Geometry check sheet. Reference: the model listing, model coordinates, mm. A direction names the side the tool comes from. Round coordinates to 2 decimals unless told otherwise and drop trailing zeros. Write each loop counter-clockwise with the first axis right and the second up, starting at its lowest first coordinate (ties: lowest second). Pieces come first, ordered by that corner, then holes. Notation, with made-up numbers: M 32.25,-11.75 L 83.25,-11.75 A12 ccw 83.25,-5.75 Z; hole C 83,20 d4. An arc over 180 degrees is marked long. Put each result on its own line as item: value. Start each with the question number.
(1) Mould release check, pull along X, two halves, no side actions. Record for faces 3 (the flat face through (-63.493, 124.331, 0.986)), 4 (the flat face through (2, 44, 0)), 5 (the cylindrical face through (48.25, 61.87, 1.01)): pulls with the +X half, pulls with the -X half, needs draft (parallel to the pull), parting line crosses it, or undercut.
(2) Material ranges on probe 1 along X at (y, z) = (14.5, 0.7); probe 2 along Y at (x, z) = (110, 1.2); probe 3 along Y at (x, z) = (91.5, 0.1), recorded low to high.
(3) Tool access check on faces 1 (the cylindrical face through (-48.25, 61.87, 1.01)), 2 (the flat face through (2, 44, 2)). Record the directions out of +Z, -Z, +X, -X, +Y, -Y that give a thin tool (end or side, any length) a straight path to the whole face; none if there is none.
(4) Section check B-B on z = 0.8. Count the separate pieces of the cut face and the enclosed holes in it, then the cut area to 3 significant figures.
(5) Gauge pin test, flat ends, axial feed: pin 1 (1 mm diameter, centred on x = -126, z = 1, fed in from +Y); pin 2 (1 mm diameter, centred on y = 107, z = 1.5, fed in from +X). Record the tip position at first contact, or that the pin passes through.
(6) Section check A-A on x = -18.5. Record the cut outline in (y, z).
from build123d import *

# Parameters (mm, degrees)
SKETCH1_W           = 20
SKETCH1_H           = 2.2
BOSS_EXTRUDE1_DEPTH = 2
FILLET1_R           = 10
SKETCH2_R           = 2.1
CUT_EXTRUDE1_DEPTH  = 5


with BuildPart() as part:
    # Sketch1 → Boss-Extrude1 (new body)
    with BuildSketch(Plane.XY):
        Polygon((125.000000001, -10.433333333), (-124.999999999, -10.433333333), (-124.999999999, 19.566666667), (-127.199999999, 19.566666667), (-127.199999999, 39.566666667), (-124.999999999, 39.566666667), (-124.999999999, 129.566666667), (-127.199999999, 129.566666667), (-127.199999999, 149.566666667), (-124.999999999, 149.566666667), (-124.999999999, 179.566666667), (-74.999999999, 179.566666667), (-50, 59.566666667), (50, 59.566666667), (75.000000001, 179.566666667), (125.000000001, 179.566666667), (125.000000001, 149.566666667), (127.200000001, 149.566666667), (127.200000001, 129.566666667), (125.000000001, 129.566666667), (125.000000001, 39.566666667), (127.200000001, 39.566666667), (127.200000001, 19.566666667), (125.000000001, 19.566666667), align=None)
        with Locations((85.000000001, -2.933333333)):
            Rectangle(SKETCH1_W, SKETCH1_H, mode=Mode.SUBTRACT)
        with Locations((-84.999999999, -2.933333333)):
            Rectangle(SKETCH1_W, SKETCH1_H, mode=Mode.SUBTRACT)
    extrude(amount=BOSS_EXTRUDE1_DEPTH)

    # Fillet1
    fillet1_edges = [part.edges().sort_by_distance(p)[0] for p in [
        (-50, 59.566666667, 1),
        (50, 59.566666667, 1),
    ]]
    fillet(fillet1_edges, radius=FILLET1_R)

    # Sketch2 → Cut-Extrude1 (cut)
    with BuildSketch(Plane.XY.offset(2)):
        with Locations((-109.999999999, 14.566666667)):
            Circle(SKETCH2_R)
        with Locations((110.000000001, 14.566666667)):
            Circle(SKETCH2_R)
        with Locations((110.000000001, 164.566666667)):
            Circle(SKETCH2_R)
        with Locations((-109.999999999, 164.566666667)):
            Circle(SKETCH2_R)
    extrude(amount=-CUT_EXTRUDE1_DEPTH, mode=Mode.SUBTRACT)


solid = part.part
Answers follow:
1. face 3: undercut
1. face 4: needs draft
1. face 5: undercut
2. probe 1: x = -125 to -112.1, -107.9 to 107.9, 112.1 to 125
2. probe 2: y = -10.43 to 12.47, 16.67 to 162.47, 166.67 to 179.57
2. probe 3: y = -10.43 to -4.03, -1.83 to 179.57
3. face 1: +Z, -Z, +Y
3. face 2: +Z, +X, -X, +Y, -Y
4. separate pieces: 1
4. enclosed holes: 6
4. area: 32,600 mm^2
5. pin 1: stops at y = 149.57
5. pin 2: stops at x = 125
6. outline: M -10.43,0 L 59.57,0 L 59.57,2 L -10.43,2 Z
